from build123d import *

# Parameters (mm, degrees)
SKETCH1_R           = 11.5
BOSS_EXTRUDE1_DEPTH = 4.5
SKETCH2_R           = 3.65
CUT_EXTRUDE1_DEPTH  = 3.1
SKETCH3_R           = 1.5
CUT_EXTRUDE2_DEPTH  = 17.556267695
CUT_EXTRUDE4_START  = -3
SKETCH4_R           = 11.5
SKETCH4_R_2         = 5.65
CUT_EXTRUDE4_DEPTH  = 3
FILLET2_R           = 0.7


with BuildPart() as part:
    # Sketch1 → Boss-Extrude1 (new body)
    with BuildSketch(Plane(origin=(0, 0, 0), x_dir=(1, 0, 0), z_dir=(0, 1, 0))):
        with Locations(Location((0, 0, 0), (0, 0, 270))):
            Circle(SKETCH1_R)
    extrude(amount=BOSS_EXTRUDE1_DEPTH)

    # Sketch2 → Cut-Extrude1 (cut)
    with BuildSketch(Plane.XZ):
        with Locations(Location((0, 0, 0), (0, 0, 270))):
            Circle(SKETCH2_R)
    extrude(amount=-CUT_EXTRUDE1_DEPTH, mode=Mode.SUBTRACT)

    # Sketch3 → Cut-Extrude2 (cut, through all)
    with BuildSketch(Plane.XZ.offset(-3.1)):
        with Locations(Location((0, 0, 0), (0, 0, 270))):
            Circle(SKETCH3_R)
    extrude(amount=-CUT_EXTRUDE2_DEPTH, mode=Mode.SUBTRACT)

    # Sketch4 → Cut-Extrude4 (cut)
    with BuildSketch(Plane(origin=(0, 4.5, 0), x_dir=(1, 0, 0), z_dir=(0, 1, 0)).offset(CUT_EXTRUDE4_START)):
        with Locations(Location((0, 0, 0), (0, 0, 270))):
            Circle(SKETCH4_R)
        with Locations(Location((0, 0, 0), (0, 0, 270))):
            Circle(SKETCH4_R_2, mode=Mode.SUBTRACT)
    extrude(amount=CUT_EXTRUDE4_DEPTH, mode=Mode.SUBTRACT)

    # Fillet2
    fillet2_edges = [part.edges().sort_by_distance(p)[0] for p in [
        (0, 1.5, -11.5),
        (0, 1.5, -5.65),
        (0, 4.5, -5.65),
    ]]
    fillet(fillet2_edges, radius=FILLET2_R)


solid = part.part
Work out the finished part from the listing and answer in its coordinate system (mm). A direction names the side the tool comes from. Give positions to 0.01 mm unless a question says otherwise; leave off trailing zeros. Write each loop counter-clockwise with the first axis right and the second up, starting at its lowest first coordinate (ties: lowest second). Pieces come first, ordered by that corner, then holes.
Q1. The part is cut by section B-B on z = 0. Give the vertices of the cut face in (x, y).
Answer:
outline: (-11.5, 0) - (-3.65, 0) - (-3.65, 3.1) - (-1.5, 3.1) - (-1.5, 4.5) - (-4.95, 4.5) arc R0.7 ccw to (-5.65, 3.8) - (-5.65, 2.2) arc R0.7 cw to (-6.35, 1.5) - (-10.8, 1.5) arc R0.7 ccw to (-11.5, 0.8) - close; (1.5, 3.1) - (3.65, 3.1) - (3.65, 0) - (11.5, 0) - (11.5, 0.8) arc R0.7 ccw to (10.8, 1.5) - (6.35, 1.5) arc R0.7 cw to (5.65, 2.2) - (5.65, 3.8) arc R0.7 ccw to (4.95, 4.5) - (1.5, 4.5) - close
Q2. Straight lines are drawn through the part: L1, parallel to X at y = 4.1, z = 0; L2, parallel to Y at x = 6.25, z = 4; L3, parallel to X at y = 1.75, z = -0.75. For each, find the intervals that lie inside material, in ascending order.
Answer:
L1: x = -5.58 to -1.5, 1.5 to 5.58
L2: y = 0 to 1.5
L3: x = -5.77 to -3.57, 3.57 to 5.77
Q3. The part is cut by section A-A on x = 0. Give the vertices of the cut face in (y, z), and give its area (3 significant figures).
Answer:
outline: (0, -11.5) - (0.8, -11.5) arc R0.7 ccw to (1.5, -10.8) - (1.5, -6.35) arc R0.7 cw to (2.2, -5.65) - (3.8, -5.65) arc R0.7 ccw to (4.5, -4.95) - (4.5, -1.5) - (3.1, -1.5) - (3.1, -3.65) - (0, -3.65) - close; (0, 3.65) - (3.1, 3.65) - (3.1, 1.5) - (4.5, 1.5) - (4.5, 4.95) arc R0.7 ccw to (3.8, 5.65) - (2.2, 5.65) arc R0.7 cw to (1.5, 6.35) - (1.5, 10.8) arc R0.7 ccw to (0.8, 11.5) - (0, 11.5) - close
area: 41.4 mm2
Q4. The part is cut by section D-D on y = 3.45. Give the vertices of the cut face in (x, z), and give its area (3 significant figures).
Answer:
outline: circle Ø11.3 at (0, 0); hole circle Ø3 at (0, 0)
area: 93.2 mm2
Q5. A tool of negligible diameter and unlimited length cuts with its end or side. For faces 4 (the face through (-1.4, 1.53, -3.37)), 5 (the face through (-5, 1.5, 5)), 6 (the face through (3, 0, -3)), from which of +Z, -Z, +X, -X, +Y, -Y can it reach the whole face along a straight path? Write none if from no direction.
Answer:
face 4: -Y
face 5: +Y
face 6: +Z, -Z, +X, -X, -Y
Q6. The part is cut by section C-C on y = 0.4. Give the vertices of the cut face in (x, z), and give its area (3 significant figures).
Answer:
outline: circle Ø23 at (0, 0); hole circle Ø7.3 at (0, 0)
area: 374 mm2
Q7. For a pull along X with two mould halves and no side action, classify faces 1 (the face through (-3.44, 2.99, -4.48)), 2 (the face through (-2, 3.1, 0)), 3 (the face through (1.2, 4.5, -1.2)) as released by +X, released by -X, zero draft, split by the parting line, or undercut.
Answer:
face 1: split by the parting line
face 2: undercut
face 3: zero draft
Q8. Given pin 1 (3.5 mm diameter, centred on x = 0.5, z = -1, fed in from -Y); pin 2 (2 mm diameter, centred on x = -4.5, z = 3.5, fed in from -Y); pin 3 (1 mm diameter, centred on x = -5.5, y = 3.5, fed in from +Z); pin 4 (2 mm diameter, centred on x = 6, z = 2, fed in from +Y), each flat-ended and moving along its own axis, determine where each tip first touches the part or whether it passes through.
Answer:
pin 1: stops at y = 3.1
pin 2: stops at y = 0
pin 3: stops at z = 2.63
pin 4: stops at y = 4.39
